Model file for the job. Use its own axes, mm. A direction names the side the tool comes from. Coordinates: 2 decimals unless noted, no trailing zeros. Write each loop counter-clockwise with the first axis right and the second up, starting at its lowest first coordinate (ties: lowest second). Pieces come first, ordered by that corner, then holes. Notation, with made-up numbers: (30.5, 85.5) -> (50.5, 85.5) arc R7 ccw to (50.5, 98.5) -> close; hole circle Ø9 at (65, 40.25). An arc over 180 degrees is marked (long way). Write item = value, one per line. Start each with the question number.
from build123d import *

# Parameters (mm, degrees)
SKETCH_1_W          = 2
SKETCH_1_H          = 37.5
SKETCH_1_W_2        = 100
SKETCH_1_H_2        = 42.5
EXTRUDE_1_DEPTH     = 2
CUT_EXTRUDE_1_REACH = 112.518
SKETCH_2_W          = 40
SKETCH_2_H          = 20


with BuildPart() as part:
    # 草图1 → 凸台-拉伸1 (new body)
    with BuildSketch(Plane(origin=(0, 0, 0), x_dir=(1, 0, 0), z_dir=(0, 1, 0))):
        with Locations((-1, 21.25)):
            Rectangle(SKETCH_1_W, SKETCH_1_H)
        with Locations((50, 21.25)):
            Rectangle(SKETCH_1_W_2, SKETCH_1_H_2)
        with Locations((101, 21.25)):
            Rectangle(SKETCH_1_W, SKETCH_1_H)
    extrude(amount=EXTRUDE_1_DEPTH)

    # 草图2 → 切除-拉伸1 (cut, up to next)
    with BuildSketch(Plane(origin=(0, 2, 0), x_dir=(1, 0, 0), z_dir=(0, 1, 0)), mode=Mode.PRIVATE) as cut_extrude_1_sk1:
        with Locations((50, 10)):
            Rectangle(SKETCH_2_W, SKETCH_2_H)
    cut_extrude_1_tool1 = extrude(cut_extrude_1_sk1.sketch, amount=-CUT_EXTRUDE_1_REACH, mode=Mode.PRIVATE) & part.part
    add(cut_extrude_1_tool1.solids().sort_by_distance((50, 2, -10))[0], mode=Mode.SUBTRACT)


solid = part.part
(1) Drop flat-ended pins along their axis: pin 1 Ø1 at (x, y) = (57, 1) entering from +Z; pin 2 Ø2 at (x, z) = (19.5, -14) entering from -Y; pin 3 Ø1 at (y, z) = (0.5, -41.5) entering from +X; pin 4 Ø1 at (y, z) = (1, -42) entering from -X. Give the stop position or say it passes through.
(2) 3-axis set-ups, long thin cutter, end or side, ignore diameter. For faces 4 (the face through (101, 1, -2.5)), 5 (the face through (0, 1, -41)), 6 (the face through (70, 1, -10)), 7 (the face through (101, 1, -40)): which of +Z, -Z, +X, -X, +Y, -Y reach the whole face in a straight line?
(3) Saw through at B-B (y = 1.45). Give the cut face in (x, z), then the cut area to 3 significant figures.
(4) Drill centre lines: line 1 along X through (y, z) = (0.75, -19); line 2 along Z through (x, y) = (67, 0.3). Where is each one in solid material? Low to high.
(5) Saw through at C-C (x = 51.5). Give the cut face in (y, z).
(6) Saw through at A-A (z = -10). Give the cut face in (x, y), then the cut area to 3 significant figures.
(7) Mould opens along X. For faces 1 (the face through (100, 1, -41)), 2 (the face through (30, 1, -10)), 3 (the face through (0, 1, -1)) say: released by +X, released by -X, zero draft, split by the parting line, or undercut.
Returned:
q1.pin_1 = -20
q1.pin_2 = 0
q1.pin_3 = 100
q1.pin_4 = 0
q2.face_4 = +Z, +X, +Y, -Y
q2.face_5 = -Z, -X, +Y, -Y
q2.face_6 = +Z, +Y, -Y
q2.face_7 = -Z, +X, +Y, -Y
q3.outline = (-2, -40) -> (0, -40) -> (0, -42.5) -> (100, -42.5) -> (100, -40) -> (102, -40) -> (102, -2.5) -> (100, -2.5) -> (100, 0) -> (70, 0) -> (70, -20) -> (30, -20) -> (30, 0) -> (0, 0) -> (0, -2.5) -> (-2, -2.5) -> close
q3.area = 3,600 mm2
q4.line_1 = -2 to 30, 70 to 102
q4.line_2 = -42.5 to -20
q5.outline = (0, -42.5) -> (2, -42.5) -> (2, -20) -> (0, -20) -> close
q6.outline = (-2, 0) -> (30, 0) -> (30, 2) -> (-2, 2) -> close; (70, 0) -> (102, 0) -> (102, 2) -> (70, 2) -> close
q6.area = 128 mm2
q7.face_1 = released by +X
q7.face_2 = undercut
q7.face_3 = released by -X
